CAD build for the part. Positions are in the model's coordinates, mm. Round coordinates to 2 decimals unless told otherwise and drop trailing zeros. Use one line per item in the form item = value. Start each with the question number.
Item 1: Pin check, flat tips, straight feed: pin 1 (10 mm diameter, centred on y = 12, z = 4.5, fed in from -X); pin 2 (10 mm diameter, centred on x = 2.5, y = -2, fed in from -Z). Stop position of each tip, or through.
Item 2: Drill centre lines: L1, parallel to Z at x = 1, y = -8; L2, parallel to X at y = 11, z = 17.5; L3, parallel to X at y = 0, z = 18. Where is each one in solid material? Low to high.
Item 3: Pull direction Y, two halves, no side cores. Call faces 1 (the flat face through (54.303, 3, 11)), 2 (the cylindrical face through (-17.37, -9.53, 12.8)), 3 (the cylindrical face through (52.88, -15.89, 13.08)): +Y half, -Y half, draft (parallel to the pull), parting line (faces both ways), or undercut.
from build123d import *

# Parameters (mm, degrees)
BOSS_EXTRUDE1_DEPTH     = 22
CUT_EXTRUDE3_DEPTH      = 64.348491393
CUT_EXTRUDE3_DEPTH_BACK = 64.348491393


with BuildPart() as part:
    # Sketch1 → Boss-Extrude1 (new body)
    with BuildSketch(Plane.XY):
        with BuildLine():
            Line((54.303030303, 17.598954753), (54.303030303, -12.396681203))
            ThreePointArc((54.303030303, -12.396681203), (52.838564209, -15.932215109), (49.303030303, -17.396681203))
            Line((49.303030303, -17.396681203), (-14.695644242, -17.396681203))
            ThreePointArc((-14.695644242, -17.396681203), (-16.816964585, -16.518001547), (-17.695644242, -14.396681203))
            Line((-17.695644242, -14.396681203), (-17.695644242, -11.306720639))
            ThreePointArc((-17.695644242, -11.306720639), (-17.35823549, -9.50110638), (-16.3915471, -7.939184142))
            add(Edge.make_bspline(
                [(-16.3915471, -7.939184142), (-0.135926549, 9.901511722), (18.69690639, 29.725737375), (49.303030303, 22.598954753)],
                knots=[0.026299547, 0.026299547, 0.026299547, 0.026299547, 1, 1, 1, 1], degree=3))
            ThreePointArc((49.303030303, 22.598954753), (52.838564209, 21.134488659), (54.303030303, 17.598954753))
        make_face()
    extrude(amount=BOSS_EXTRUDE1_DEPTH)

    # Sketch3 → Cut-Extrude3 (cut, two sides: drawn at the far end of the back side and taken through both)
    with BuildSketch(Plane(origin=(0, 0, 0), x_dir=(0, 0, -1), z_dir=(1, 0, 0)).offset(-CUT_EXTRUDE3_DEPTH_BACK)):
        Polygon((12.434475201, 127.254636362), (0, 24.087595181), (-5, -17.396681203), (-17.434475201, -120.563722385), (188.899607163, -145.432672786), (218.768557564, 102.385685961), align=None)
    extrude(amount=CUT_EXTRUDE3_DEPTH + CUT_EXTRUDE3_DEPTH_BACK, mode=Mode.SUBTRACT)


solid = part.part
Determined:
q1.pin_1 = -1.79
q1.pin_2 = 2.54
q2.L1 = 3.87 to 22
q2.L2 = 2.91 to 54.3
q2.L3 = -8.99 to 54.3
q3.face_1 = draft
q3.face_2 = +Y half
q3.face_3 = -Y half
